```python
from build123d import *

# Parameters (mm, degrees)
SKETCH1_R           = 27.5
SKETCH1_R_2         = 17.5
BOSS_EXTRUDE1_DEPTH = 5
SKETCH2_W           = 120
SKETCH2_H           = 6
BOSS_EXTRUDE2_DEPTH = 10
SKETCH3_W           = 5
SKETCH3_H           = 3
CUT_EXTRUDE2_DEPTH  = 140
SKETCH4_W           = 5
SKETCH4_H           = 3
CUT_EXTRUDE3_DEPTH  = 10
CHAMFER2_SIZE       = 5
SKETCH5_W           = 5
SKETCH5_H           = 3
CUT_EXTRUDE4_DEPTH  = 110
CHAMFER3_SIZE       = 5
SKETCH6_R           = 3.25
CUT_EXTRUDE5_DEPTH  = 110


# Some blends are built 0.0001 mm under size
with BuildPart() as part:
    # Sketch1 → Boss-Extrude1 (new body)
    with BuildSketch(Plane.XY):
        Circle(SKETCH1_R)
        Circle(SKETCH1_R_2, mode=Mode.SUBTRACT)
    extrude(amount=BOSS_EXTRUDE1_DEPTH)

    # Sketch2 → Boss-Extrude2 (add)
    with BuildSketch(Plane.XY.offset(5)):
        with Locations((77.5, 0)):
            Rectangle(SKETCH2_W, SKETCH2_H)
    extrude(amount=-BOSS_EXTRUDE2_DEPTH)

    # Sketch3 → Cut-Extrude2 (cut)
    with BuildSketch(Plane.ZY.offset(-17.5)):
        with Locations((-2.5, -1.5)):
            Rectangle(SKETCH3_W, SKETCH3_H)
    extrude(amount=-CUT_EXTRUDE2_DEPTH, mode=Mode.SUBTRACT)

    # Sketch4 → Cut-Extrude3 (cut)
    with BuildSketch(Plane.ZY.offset(-17.5)):
        with Locations((-2.5, 1.5)):
            Rectangle(SKETCH4_W, SKETCH4_H)
    extrude(amount=-CUT_EXTRUDE3_DEPTH, mode=Mode.SUBTRACT)

    # Chamfer2
    chamfer2_edges = [part.edges().sort_by_distance(p)[0] for p in [
        (27.5, 1.5, -5),
    ]]
    chamfer(chamfer2_edges, length=CHAMFER2_SIZE - 0.0001)  # a hair under: the kernel refuses the full size

    # Sketch5 → Cut-Extrude4 (cut)
    with BuildSketch(Plane(origin=(137.5, 0, 0), x_dir=(0, 0, -1), z_dir=(1, 0, 0))):
        with Locations((-2.5, -1.5)):
            Rectangle(SKETCH5_W, SKETCH5_H)
    extrude(amount=-CUT_EXTRUDE4_DEPTH, mode=Mode.SUBTRACT)

    # Chamfer3
    # the kernel refuses this chamfer: 5.650095031, 5 mm, written as the material it adds along each edge
    with BuildSketch(Plane(origin=(27.335873866, 3, 5), x_dir=(1, 0, 0), z_dir=(0, 0, -1))) as chamfer3_piece_1_section:
        with BuildLine():
            Line((CHAMFER3_SIZE, 0), (-1.545806391, -6.545806391))
            ThreePointArc((-1.545806391, -6.545806391), (-0.594506403, -3.414769383), (0, 0))
            Line((0, 0), (CHAMFER3_SIZE, 0))
        make_face()
    chamfer3_piece_1 = extrude(amount=5, mode=Mode.PRIVATE)
    chamfer3_piece_1 = split(chamfer3_piece_1, bisect_by=Plane(origin=(27.5, 3, 5), z_dir=(1, 0, 0)), keep=Keep.TOP, mode=Mode.PRIVATE)
    add(chamfer3_piece_1)
    with BuildSketch(Plane(origin=(27.335873866, 3, 5), x_dir=(1, 0, 0), z_dir=(0, 0, -1))) as chamfer3_piece_2_section:
        with BuildLine():
            Line((CHAMFER3_SIZE, 0), (-1.545806391, -6.545806391))
            ThreePointArc((-1.545806391, -6.545806391), (-0.594506403, -3.414769383), (0, 0))
            Line((0, 0), (CHAMFER3_SIZE, 0))
        make_face()
    chamfer3_piece_2 = extrude(amount=5, mode=Mode.PRIVATE)
    chamfer3_piece_2 = split(chamfer3_piece_2, bisect_by=Plane(origin=(24.917886933, 3, 2.582013067), z_dir=(0.7071067811865478, 0, 0.7071067811865472)), keep=Keep.TOP, mode=Mode.PRIVATE)
    chamfer3_piece_2 = split(chamfer3_piece_2, bisect_by=Plane(origin=(27.5, 3, 5), z_dir=(-1, 0, 0)), keep=Keep.TOP, mode=Mode.PRIVATE)
    add(chamfer3_piece_2)
    with BuildSketch(Plane(origin=(27.335873866, 3, 5), x_dir=(1, 0, 0), z_dir=(0, 0, -1))) as chamfer3_piece_3_section:
        with BuildLine():
            Line((CHAMFER3_SIZE, 0), (-1.545806391, -6.545806391))
            ThreePointArc((-1.545806391, -6.545806391), (-0.594506403, -3.414769383), (0, 0))
            Line((0, 0), (CHAMFER3_SIZE, 0))
        make_face()
    chamfer3_piece_3 = extrude(amount=22.297831984, mode=Mode.PRIVATE)
    chamfer3_piece_3 = split(chamfer3_piece_3, bisect_by=Plane(origin=(24.917886933, 3, 2.582013067), z_dir=(0.7071067811865478, 0, 0.7071067811865472)), keep=Keep.TOP, mode=Mode.PRIVATE)
    chamfer3_piece_3 = split(chamfer3_piece_3, bisect_by=Plane(origin=(27.335873866, 3, 0), z_dir=(0, 0, -1)), keep=Keep.TOP, mode=Mode.PRIVATE)
    add(chamfer3_piece_3)
    with BuildSketch(Plane(origin=(27.335873866, 3, 5), x_dir=(1, 0, 0), z_dir=(0, 0, -1))) as chamfer3_piece_4_section:
        with BuildLine():
            Line((CHAMFER3_SIZE, 0), (-1.545806391, -6.545806391))
            ThreePointArc((-1.545806391, -6.545806391), (-0.594506403, -3.414769383), (0, 0))
            Line((0, 0), (CHAMFER3_SIZE, 0))
        make_face()
    chamfer3_piece_4 = extrude(amount=5, mode=Mode.PRIVATE)
    chamfer3_piece_4 = split(chamfer3_piece_4, bisect_by=Plane(origin=(24.917886933, 3, 2.582013067), z_dir=(-0.7071067811865478, 0, -0.7071067811865472)), keep=Keep.TOP, mode=Mode.PRIVATE)
    add(chamfer3_piece_4)

    # Sketch6 → Cut-Extrude5 (cut)
    with BuildSketch(Plane.XZ):
        with Locations(Location((97.5, 0, 0), (0, 0, 270))):
            Circle(SKETCH6_R)
    extrude(amount=-CUT_EXTRUDE5_DEPTH, mode=Mode.SUBTRACT)


solid = part.part
```
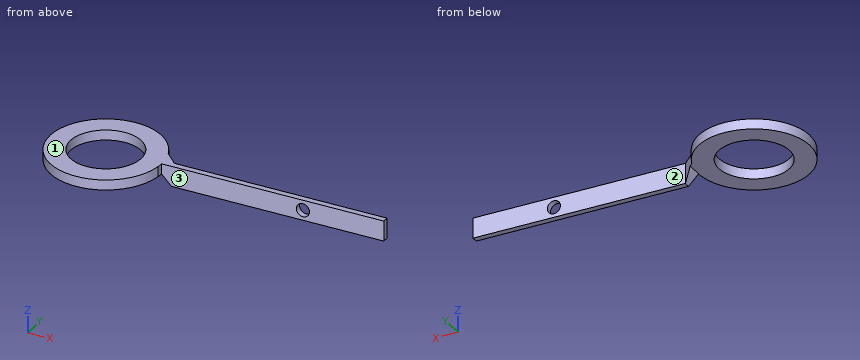
For this review, take the finished solid that the model builds, in its own axes (mm). Face numbers are marked on the shaded views. A direction names the side the tool comes from. Coordinates: 2 decimals unless noted, no trailing zeros. Order: outer loops, then holes, each group sorted by start corner. A loop starts at its lowest first (then second) coordinate and runs counter-clockwise, first axis right, second up. Notation, with made-up numbers: (-39.75, 36) -> (-22.75, 36) arc R16 ccw to (-22.75, 50) -> close; hole circle Ø2 at (-10, -26). An arc over 180 degrees is marked (long way). Answer as CSV lines item,"result".
Q1. We need section A-A (x = 0). State the section outline as (y, z) points, plus the area to 3 significant figures.
Model answer:
outline,"(-27.5, 0) -> (-17.5, 0) -> (-17.5, 5) -> (-27.5, 5) -> close; (17.5, 0) -> (27.5, 0) -> (27.5, 5) -> (17.5, 5) -> close"
area,"100 mm2"
Q2. Wall thickness on line 1 along Y through (x, z) = (0, 2.65); line 2 along Y through (x, z) = (127, -1); line 3 along Z through (x, y) = (17.5, -5.5): over which ranges is each line inside the solid? List them lowest first. Write a range as [from, to].
Model answer:
line 1,"y = [-27.5, -17.5], [17.5, 27.5]"
line 2,"y = [0, 3]"
line 3,"z = [0, 5]"
Q3. Clearance check with flat-ended pins moving along their axes: pin 1 Ø5 at (y, z) = (-17.5, -1) entering from +X; pin 2 Ø6 at (x, z) = (97.5, 0) entering from +Y; pin 3 Ø5 at (x, z) = (75, 2) entering from -Y; pin 4 Ø1.5 at (y, z) = (-9.5, 1.5) entering from -X. State where each tip first meets the part, or that it passes through.
Model answer:
pin 1,"stops at x = 22.91"
pin 2,"passes through"
pin 3,"stops at y = 0"
pin 4,"stops at x = -26.07"
Q4. For the marked faces 1, 2 and 3, list the 3-axis set-ups (+Z, -Z, +X, -X, +Y, -Y) from which the entire face can be reached by the end or side of a thin tool; tool diameter is ignored.
Model answer:
face 1,"+Z, +X, -X, +Y, -Y"
face 2,"+Z, -Z, +X, +Y"
face 3,"+Z, -Z, +X, -Y"
Q5. We need section D-D (x = 39). State the section outline as (y, z) points, plus the area to 3 significant figures.
Model answer:
outline,"(0, -5) -> (3, -5) -> (3, 5) -> (0, 5) -> close"
area,"30.0 mm2"
Q6. We need section B-B (z = 1.5). State the section outline as (x, y) points.
Model answer:
outline,"(25.79, 9.55) arc R27.5 ccw (long way) to (27.34, -3) -> (27.5, -3) -> (27.5, 0) -> (94.62, 0) -> (94.62, 3) -> (32.34, 3) -> close; (100.38, 0) -> (137.5, 0) -> (137.5, 3) -> (100.38, 3) -> close; hole circle Ø35 at (0, 0)"
Q7. We need section C-C (y = -10.5). State the section outline as (x, z) points.
Model answer:
outline,"(-25.42, 0) -> (-14, 0) -> (-14, 5) -> (-25.42, 5) -> close; (14, 0) -> (25.42, 0) -> (25.42, 5) -> (14, 5) -> close"
